The model under review builds one solid part; all positions refer to its coordinate system, in mm. Coordinates: 2 decimals unless noted, no trailing zeros. Order: outer loops, then holes, each group sorted by start corner. A loop starts at its lowest first (then second) coordinate and runs counter-clockwise, first axis right, second up.
```python
from build123d import *

# Parameters (mm, degrees)
SKETCH1_W           = 26
SKETCH1_H           = 1
BOSS_EXTRUDE1_DEPTH = 21
SKETCH2_W           = 2
SKETCH2_H           = 1.5
CUT_EXTRUDE1_DEPTH  = 1
CUT_EXTRUDE3_REACH  = 26.718
SKETCH3_R           = 3.75


with BuildPart() as part:
    # Sketch1 → Boss-Extrude1 (new body)
    with BuildSketch(Plane(origin=(0, 0, 0), x_dir=(1, 0, 0), z_dir=(0, 1, 0))):
        Rectangle(SKETCH1_W, SKETCH1_H)
    extrude(amount=BOSS_EXTRUDE1_DEPTH)

    # Sketch2 → Cut-Extrude1 (cut)
    with BuildSketch(Plane.XY.offset(0.5)):
        with Locations((-4.5, 17.25)):
            Rectangle(SKETCH2_W, SKETCH2_H)
        with Locations((-9, 17.25)):
            Rectangle(SKETCH2_W, SKETCH2_H)
        with Locations((0, 17.25)):
            Rectangle(SKETCH2_W, SKETCH2_H)
        with Locations((4.5, 17.25)):
            Rectangle(SKETCH2_W, SKETCH2_H)
        with Locations((9, 17.25)):
            Rectangle(SKETCH2_W, SKETCH2_H)
        with Locations((-9, 13.883333)):
            Rectangle(SKETCH2_W, SKETCH2_H)
        with Locations((-4.5, 13.883333)):
            Rectangle(SKETCH2_W, SKETCH2_H)
        with Locations((0, 13.883333)):
            Rectangle(SKETCH2_W, SKETCH2_H)
        with Locations((4.5, 13.883333)):
            Rectangle(SKETCH2_W, SKETCH2_H)
        with Locations((9, 13.883333)):
            Rectangle(SKETCH2_W, SKETCH2_H)
        with Locations((-9, 10.516666)):
            Rectangle(SKETCH2_W, SKETCH2_H)
        with Locations((-4.5, 10.516666)):
            Rectangle(SKETCH2_W, SKETCH2_H)
        with Locations((0, 10.516666)):
            Rectangle(SKETCH2_W, SKETCH2_H)
        with Locations((4.5, 10.516666)):
            Rectangle(SKETCH2_W, SKETCH2_H)
        with Locations((9, 10.516666)):
            Rectangle(SKETCH2_W, SKETCH2_H)
        with Locations((-9, 7.149999)):
            Rectangle(SKETCH2_W, SKETCH2_H)
        with Locations((-4.5, 7.149999)):
            Rectangle(SKETCH2_W, SKETCH2_H)
        with Locations((0, 7.149999)):
            Rectangle(SKETCH2_W, SKETCH2_H)
        with Locations((4.5, 7.149999)):
            Rectangle(SKETCH2_W, SKETCH2_H)
        with Locations((9, 7.149999)):
            Rectangle(SKETCH2_W, SKETCH2_H)
        with Locations((-9, 3.783332)):
            Rectangle(SKETCH2_W, SKETCH2_H)
        with Locations((-4.5, 3.783332)):
            Rectangle(SKETCH2_W, SKETCH2_H)
        with Locations((0, 3.783332)):
            Rectangle(SKETCH2_W, SKETCH2_H)
        with Locations((4.5, 3.783332)):
            Rectangle(SKETCH2_W, SKETCH2_H)
        with Locations((9, 3.783332)):
            Rectangle(SKETCH2_W, SKETCH2_H)
    extrude(amount=-CUT_EXTRUDE1_DEPTH, mode=Mode.SUBTRACT)

    # Sketch3 → Cut-Extrude3 (cut, up to next)
    with BuildSketch(Plane.XY.offset(0.5), mode=Mode.PRIVATE) as cut_extrude3_sk1:
        with Locations((0, 10.5)):
            Circle(SKETCH3_R)
    cut_extrude3_tool1 = extrude(cut_extrude3_sk1.sketch, amount=-CUT_EXTRUDE3_REACH, mode=Mode.PRIVATE) & part.part
    add(cut_extrude3_tool1.solids().sort_by_distance((0, 10.5, 0.5))[0], mode=Mode.SUBTRACT)


solid = part.part
```
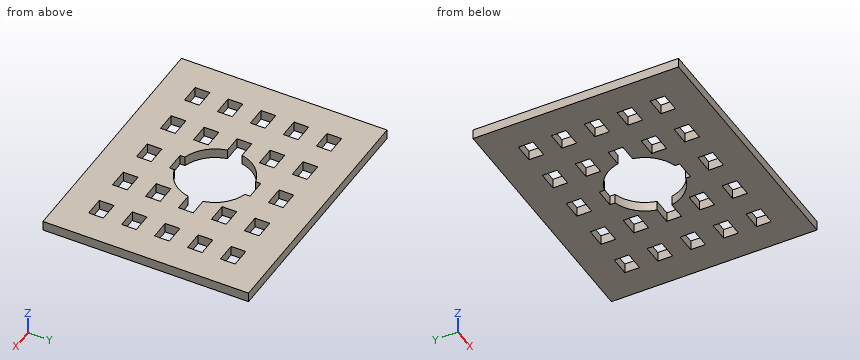
(1) We need section B-B, the plane x = 8.75. Write out the cut boundary in (y, z).
A:
outline: (0, -0.5) - (3.03, -0.5) - (3.03, 0.5) - (0, 0.5) - close; (4.53, -0.5) - (6.4, -0.5) - (6.4, 0.5) - (4.53, 0.5) - close; (7.9, -0.5) - (9.77, -0.5) - (9.77, 0.5) - (7.9, 0.5) - close; (11.27, -0.5) - (13.13, -0.5) - (13.13, 0.5) - (11.27, 0.5) - close; (14.63, -0.5) - (16.5, -0.5) - (16.5, 0.5) - (14.63, 0.5) - close; (18, -0.5) - (21, -0.5) - (21, 0.5) - (18, 0.5) - close
(2) We need section A-A, the plane y = 17.25. Write out the cut boundary in (x, z), and give its area (3 significant figures).
A:
outline: (-13, -0.5) - (-10, -0.5) - (-10, 0.5) - (-13, 0.5) - close; (-8, -0.5) - (-5.5, -0.5) - (-5.5, 0.5) - (-8, 0.5) - close; (-3.5, -0.5) - (-1, -0.5) - (-1, 0.5) - (-3.5, 0.5) - close; (1, -0.5) - (3.5, -0.5) - (3.5, 0.5) - (1, 0.5) - close; (5.5, -0.5) - (8, -0.5) - (8, 0.5) - (5.5, 0.5) - close; (10, -0.5) - (13, -0.5) - (13, 0.5) - (10, 0.5) - close
area: 16.0 mm2
(3) We need section C-C, the plane z = 0. Count the separate pieces of the cut face and the enclosed holes in it, and give its area (3 significant figures).
A:
separate pieces: 1
enclosed holes: 21
area: 435 mm2
(4) Wall thickness on probe 1 along Y at (x, z) = (-4, -0.3); probe 2 along X at (y, z) = (10.5, 0.4); probe 3 along X at (y, z) = (3.25, 0.3): over which ranges is each line inside the solid? List them lowest first.
A:
probe 1: y = 0 to 3.03, 4.53 to 6.4, 7.9 to 9.77, 11.27 to 13.13, 14.63 to 16.5, 18 to 21
probe 2: x = -13 to -10, -8 to -5.5, 5.5 to 8, 10 to 13
probe 3: x = -13 to -10, -8 to -5.5, -3.5 to -1, 1 to 3.5, 5.5 to 8, 10 to 13
